Can you work these out from the model? Positions are in its coordinate system, mm. A direction names the side the tool comes from. Give positions to 0.01 mm unless a question says otherwise; leave off trailing zeros. Loops run counter-clockwise (first coordinate to the right, second up) from the corner with the lowest first, then second, coordinate; pieces in that order, holes last. Notation, with made-up numbers: M 60,-27.75 L 105,-27.75 A22 ccw 105,9.25 Z; hole C 3,-19.75 d10. An arc over 180 degrees is marked long. Answer as a JSON object with one key per item and string values.
```python
from build123d import *

# Parameters (mm, degrees)
F0_W     = 1.5
F0_H     = 10.375
F0_H_2   = 1.5
F0_W_2   = 7.9
F0_H_3   = 7.9
F0_W_3   = 7.875
F0_W_4   = 1.360903731
F0_W_5   = 6.539096269
F1_DEPTH = 13.5


with BuildPart() as f1:
    # F0 (on Top) → F1 (new body)
    with BuildSketch(Plane.XY):
        with Locations((-18.025, 15.3375)):
            Rectangle(F0_W, F0_H)
        with Locations((-18.025, 9.4)):
            Rectangle(F0_W, F0_H_2)
        with Locations((-22.725, 9.4)):
            Rectangle(F0_W_2, F0_H_2)
        with Locations((-18.025, 4.7)):
            Rectangle(F0_W, F0_H_3)
        with Locations((-18.025, 0)):
            Rectangle(F0_W, F0_H_2)
        with Locations((-22.725, 0)):
            Rectangle(F0_W_2, F0_H_2)
        with Locations((-18.025, -4.7)):
            Rectangle(F0_W, F0_H_3)
        with Locations((-18.025, -9.4)):
            Rectangle(F0_W, F0_H_2)
        with Locations((-22.725, -9.4)):
            Rectangle(F0_W_2, F0_H_2)
        with Locations((-18.025, -15.3375)):
            Rectangle(F0_W, F0_H)
        with Locations((-13.3375, -9.4)):
            Rectangle(F0_W_3, F0_H_2)
        with Locations((-8.65, -9.4)):
            Rectangle(F0_W, F0_H_2)
        with Locations((-8.65, -4.7)):
            Rectangle(F0_W, F0_H_3)
        with Locations((-8.65, 0)):
            Rectangle(F0_W, F0_H_2)
        with Locations((-13.3375, 0)):
            Rectangle(F0_W_3, F0_H_2)
        with Locations((-8.65, -15.3375)):
            Rectangle(F0_W, F0_H)
        with Locations((-8.65, 15.3375)):
            Rectangle(F0_W, F0_H)
        with Locations((-8.65, 9.4)):
            Rectangle(F0_W, F0_H_2)
        with Locations((-8.65, 4.7)):
            Rectangle(F0_W, F0_H_3)
        with Locations((-13.3375, 9.4)):
            Rectangle(F0_W_3, F0_H_2)
        with Locations((-3.95, 9.4)):
            Rectangle(F0_W_2, F0_H_2)
        with Locations((0.75, 9.4)):
            Rectangle(F0_W, F0_H_2)
        with Locations((0.75, 15.3375)):
            Rectangle(F0_W, F0_H)
        with Locations((0.75, 4.7)):
            Rectangle(F0_W, F0_H_3)
        with Locations((-3.95, 0)):
            Rectangle(F0_W_2, F0_H_2)
        with Locations((0.75, 0)):
            Rectangle(F0_W, F0_H_2)
        with Locations((0.75, -4.7)):
            Rectangle(F0_W, F0_H_3)
        with Locations((0.75, -9.4)):
            Rectangle(F0_W, F0_H_2)
        with Locations((-3.95, -9.4)):
            Rectangle(F0_W_2, F0_H_2)
        with Locations((0.75, -15.3375)):
            Rectangle(F0_W, F0_H)
        with Locations((5.45, -9.4)):
            Rectangle(F0_W_2, F0_H_2)
        with Locations((10.15, -15.3375)):
            Rectangle(F0_W, F0_H)
        with Locations((19.4554518655, -15.3375)):
            Rectangle(F0_W_4, F0_H)
        with Locations((23.4054518655, -9.4)):
            Rectangle(F0_W_5, F0_H_2)
        with Locations((14.8375, -9.4)):
            Rectangle(F0_W_3, F0_H_2)
        with Locations((19.4554518655, -9.4)):
            Rectangle(F0_W_4, F0_H_2)
        with Locations((10.15, -9.4)):
            Rectangle(F0_W, F0_H_2)
        with Locations((10.15, -4.7)):
            Rectangle(F0_W, F0_H_3)
        with Locations((19.4554518655, -4.7)):
            Rectangle(F0_W_4, F0_H_3)
        with Locations((19.4554518655, 0)):
            Rectangle(F0_W_4, F0_H_2)
        with Locations((14.8375, 0)):
            Rectangle(F0_W_3, F0_H_2)
        with Locations((10.15, 0)):
            Rectangle(F0_W, F0_H_2)
        with Locations((5.45, 0)):
            Rectangle(F0_W_2, F0_H_2)
        with Locations((19.4554518655, 4.7)):
            Rectangle(F0_W_4, F0_H_3)
        with Locations((10.15, 4.7)):
            Rectangle(F0_W, F0_H_3)
        with Locations((23.4054518655, 0)):
            Rectangle(F0_W_5, F0_H_2)
        with Locations((23.4054518655, 9.4)):
            Rectangle(F0_W_5, F0_H_2)
        with Locations((14.8375, 9.4)):
            Rectangle(F0_W_3, F0_H_2)
        with Locations((19.4554518655, 9.4)):
            Rectangle(F0_W_4, F0_H_2)
        with Locations((19.4554518655, 15.3375)):
            Rectangle(F0_W_4, F0_H)
        with Locations((10.15, 15.3375)):
            Rectangle(F0_W, F0_H)
        with Locations((10.15, 9.4)):
            Rectangle(F0_W, F0_H_2)
        with Locations((5.45, 9.4)):
            Rectangle(F0_W_2, F0_H_2)
    extrude(amount=F1_DEPTH)


solid = f1.part
```
1) Suppose I cut it at C-C, the plane z = 3.5. Give the number of separate pieces and of enclosed holes in the cut face, and give its area (3 significant figures).
Answer list:
{"separate pieces": "1", "enclosed holes": "8", "area": "509 mm^2"}
2) If we mould it in two halves opening along X, with no side actions, what happens to faces 1 (the flat face through (-17.275, -5, 7)), 2 (the flat face through (-9.4, 15, 7)), 3 (the flat face through (-18.775, -15, 7)), 4 (the flat face through (23, 0.75, 7))? For each: +X half, -X half, draft (parallel to the pull), parting line (faces both ways), or undercut.
Answer list:
{"face 1": "undercut", "face 2": "undercut", "face 3": "-X half", "face 4": "draft"}
3) Please list where these lines run through material, in increasing order: line 1 along Y through (x, z) = (-24, 3.5); line 2 along X through (y, z) = (-18, 9) (3 decimals). Write a range as from..to.
Answer list:
{"line 1": "-10.15..-8.65, -0.75..0.75, 8.65..10.15", "line 2": "-18.775..-17.275, -9.4..-7.9, 0..1.5, 9.4..10.9, 18.775..20.136"}
4) Suppose I cut it at A-A, the plane y = -3.5. Write out the boundary of the cut face in (x, z) (3 decimals), and give its area (3 significant figures).
Answer list:
{"outline": "M -18.775,0 L -17.275,0 L -17.275,13.5 L -18.775,13.5 Z; M -9.4,0 L -7.9,0 L -7.9,13.5 L -9.4,13.5 Z; M 0,0 L 1.5,0 L 1.5,13.5 L 0,13.5 Z; M 9.4,0 L 10.9,0 L 10.9,13.5 L 9.4,13.5 Z; M 18.775,0 L 20.136,0 L 20.136,13.5 L 18.775,13.5 Z", "area": "99.4 mm^2"}
5) For faces 5 (the flat face through (1.5, -5, 7)), 6 (the flat face through (23, -10.15, 7)), 7 (the flat face through (-23, -8.65, 7)), 8 (the flat face through (-17.275, -15, 7)), which set-ups out of +Z, -Z, +X, -X, +Y, -Y let a thin tool reach every point of the face, with its end or its side?
Answer list:
{"face 5": "+Z, -Z", "face 6": "+Z, -Z, +X, -Y", "face 7": "+Z, -Z, -X", "face 8": "+Z, -Z, -Y"}
6) Suppose I cut it at B-B, the plane x = -23. Write out the boundary of the cut face in (y, z).
Answer list:
{"outline": "M -10.15,0 L -8.65,0 L -8.65,13.5 L -10.15,13.5 Z; M -0.75,0 L 0.75,0 L 0.75,13.5 L -0.75,13.5 Z; M 8.65,0 L 10.15,0 L 10.15,13.5 L 8.65,13.5 Z"}
7) Will these pins go through, and if not, where does the flat tip stop? pin 1 Ø5 at (y, z) = (-14.5, 10) entering from +X; pin 2 Ø4 at (x, z) = (-14.5, 5.5) entering from +Y; pin 3 Ø2 at (x, y) = (6.5, -15) entering from +Z; pin 4 Ø5 at (x, z) = (-12, 11.5) entering from -Y.
Answer list:
{"pin 1": "x = 20.14", "pin 2": "y = 10.15", "pin 3": "through", "pin 4": "y = -10.15"}
